```python
from build123d import *

# Parameters (mm, degrees)
SKETCH1_W           = 50
SKETCH1_H           = 22
BOSS_EXTRUDE1_DEPTH = 0.1
SKETCH2_W           = 55
SKETCH2_H           = 5
BOSS_EXTRUDE2_DEPTH = 0.05
CIRPATTERN1_COUNT   = 2


with BuildPart() as part:
    # Sketch1 → Boss-Extrude1 (new body)
    with BuildSketch(Plane(origin=(0, 0, 0), x_dir=(1, 0, 0), z_dir=(0, 1, 0))):
        Rectangle(SKETCH1_W, SKETCH1_H)
    extrude(amount=BOSS_EXTRUDE1_DEPTH)

    # Sketch2 → Boss-Extrude2 (add)
    with BuildSketch(Plane(origin=(0, 0.1, 0), x_dir=(1, 0, 0), z_dir=(0, 1, 0))):
        with Locations((2.5, 8.5)):
            Rectangle(SKETCH2_W, SKETCH2_H)
    extrude(amount=BOSS_EXTRUDE2_DEPTH)


with BuildPart() as cirpattern1_1:
    # CirPattern1: pattern copy
    add(part.part.rotate(Axis((0, 0, 0), (1, 0, 0)), 1 * 360 / CIRPATTERN1_COUNT))

    # Combine2: union part
    add(part.part)


solid = cirpattern1_1.part
```
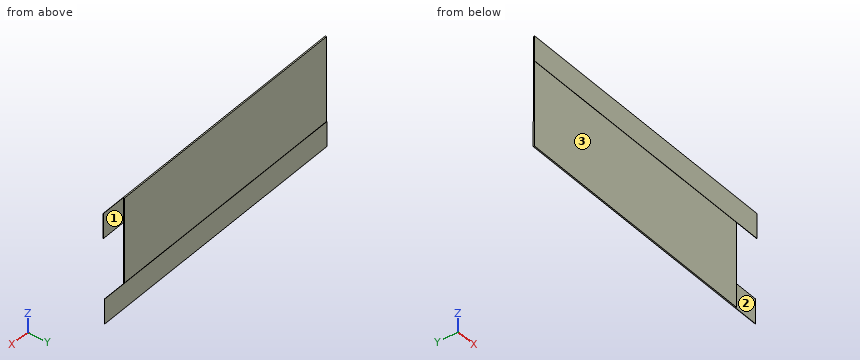
Input: part model. Units: mm. Frame: model coordinates. Face numbers are marked on the shaded views. A direction names the side the tool comes from. Give positions to 0.01 mm unless a question says otherwise; leave off trailing zeros. Order: outer loops, then holes, each group sorted by start corner. A loop starts at its lowest first (then second) coordinate and runs counter-clockwise, first axis right, second up. Notation, with made-up numbers: M -39,-35.5 L 2,-35.5 A21 cw 2,-25.5 Z; hole C -38.5,-28.75 d5. An arc over 180 degrees is marked long. One line per question, with ' | ' between items.
1) Section B-B on z = -9.25. Output: boundary loops of the cut face in (x, y), and give its area (4 significant figures).
Filled in:
outline: M -25,-0.1 L 25,-0.1 L 25,0.1 L 30,0.1 L 30,0.15 L -25,0.15 Z | area: 12.75 mm2
2) Section C-C on y = 0. Output: boundary loops of the cut face in (x, z), and give its area (3 significant figures).
Filled in:
outline: M -25,-11 L 25,-11 L 25,11 L -25,11 Z | area: 1,100 mm2
3) Access query for the marked faces 1, 2 and 3. Directions: +Z, -Z, +X, -X, +Y, -Y. A direction counts if a zero-diameter tool reaches every point of the face in a straight line with its end or side. Return the directions, or none.
Filled in:
face 1: +Z, -Z, +X, +Y | face 2: +Z, -Z, +X, -Y | face 3: -Z, +X, -X, -Y
4) Section D-D on z = -4.5. Output: boundary loops of the cut face in (x, y), and give its area (3 significant figures).
Filled in:
outline: M -25,-0.1 L 25,-0.1 L 25,0.1 L -25,0.1 Z | area: 10.0 mm2
5) Section A-A on x = -11. Output: boundary loops of the cut face in (y, z).
Filled in:
outline: M -0.15,6 L -0.1,6 L -0.1,-11 L 0.15,-11 L 0.15,-6 L 0.1,-6 L 0.1,11 L -0.15,11 Z
6) Ray query, L1, parallel to Y at x = 19, z = -0.5; L2, parallel to X at y = 0.05, z = 10; L3, parallel to Y at x = -18.5, z = -6.25. Return the intervals inside material, ascending.
Filled in:
L1: y = -0.1 to 0.1 | L2: x = -25 to 25 | L3: y = -0.1 to 0.15
7) Contact query for flat-ended pins moving along their axis: P1, Ø6, axis at x = -12.5, z = -1.5, coming from the +Y side; P2, Ø5.5, axis at x = 28, z = 9, coming from the +Y side; P3, Ø8.5, axis at x = -10.5, z = 1, coming from the -Y side. Output: stop coordinate, or through.
Filled in:
P1: stops at y = 0.1 | P2: stops at y = -0.1 | P3: stops at y = -0.1
